CAD build for the part. Positions are in the model's coordinates, mm. Face numbers are marked on the shaded views. A direction names the side the tool comes from. Coordinates: 2 decimals unless noted, no trailing zeros. Write each loop counter-clockwise with the first axis right and the second up, starting at its lowest first coordinate (ties: lowest second). Pieces come first, ordered by that corner, then holes. Notation, with made-up numbers: (87.5, 87.25) -> (91.5, 87.25) arc R15 cw to (91.5, 113.25) -> close; hole circle Ø2 at (73, 63). An arc over 180 degrees is marked (long way). Answer as CSV lines item,"result".
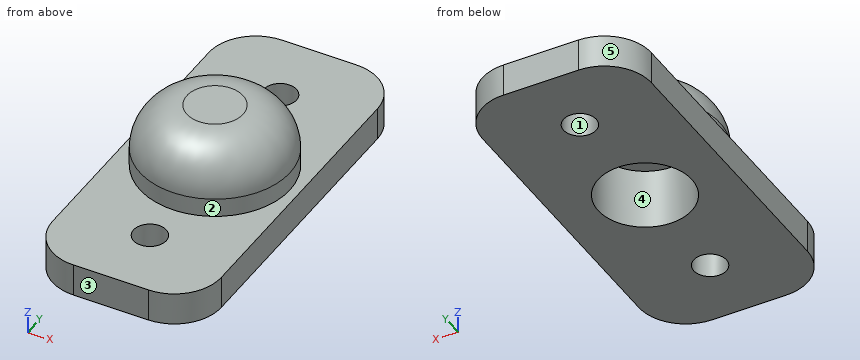
```python
from build123d import *

# Parameters (mm, degrees)
SKETCH1_W           = 18
SKETCH1_H           = 40
SKETCH1_R           = 1.75
BOSS_EXTRUDE1_DEPTH = 3.5
SKETCH2_R           = 8
BOSS_EXTRUDE2_DEPTH = 7
SKETCH3_R           = 5
CUT_EXTRUDE1_DEPTH  = 6.5
FILLET1_R           = 5


with BuildPart() as part:
    # Sketch1 → Boss-Extrude1 (new body)
    with BuildSketch(Plane.XY):
        with Locations((-6.970291657, 8.814124101)):
            Rectangle(SKETCH1_W, SKETCH1_H)
        with Locations((-6.970291657, 21.314124101)):
            Circle(SKETCH1_R, mode=Mode.SUBTRACT)
        with Locations((-6.970291657, -3.685875899)):
            Circle(SKETCH1_R, mode=Mode.SUBTRACT)
    extrude(amount=BOSS_EXTRUDE1_DEPTH)

    # Sketch2 → Boss-Extrude2 (add)
    with BuildSketch(Plane.XY.offset(3.5)):
        with Locations((-6.970291657, 8.814124101)):
            Circle(SKETCH2_R)
    extrude(amount=BOSS_EXTRUDE2_DEPTH)

    # Sketch3 → Cut-Extrude1 (cut)
    with BuildSketch(Plane(origin=(0, 0, 0), x_dir=(-1, 0, 0), z_dir=(0, 0, -1))):
        with Locations((6.970291657, 8.814124101)):
            Circle(SKETCH3_R)
    extrude(amount=-CUT_EXTRUDE1_DEPTH, mode=Mode.SUBTRACT)

    # Fillet1
    fillet1_edges = [part.edges().sort_by_distance(p)[0] for p in [
        (-14.970291657, 8.814124101, 10.5),
        (-15.970291657, 28.814124101, 1.75),
        (2.029708343, 28.814124101, 1.75),
        (2.029708343, -11.185875899, 1.75),
        (-15.970291657, -11.185875899, 1.75),
    ]]
    fillet(fillet1_edges, radius=FILLET1_R)


solid = part.part
```
Item 1: Flat gauge pins, fed straight in: pin 1 (4.5 mm diameter, centred on x = -6.97, y = -3.69, fed in from +Z); pin 2 (9 mm diameter, centred on x = -10, y = 16.5, fed in from +Z); pin 3 (1 mm diameter, centred on x = -13, z = 3.5, fed in from +Y); pin 4 (1 mm diameter, centred on y = 0.5, z = 9, fed in from -X). Where does each tip first touch, or does it go through?
Answer below:
pin 1,"stops at z = 3.5"
pin 2,"stops at z = 10.44"
pin 3,"stops at y = 28.57"
pin 4,"passes through"
Item 2: Saw through at A-A on z = 2.75. Give the cut face in (x, y), and give its area (3 significant figures).
Answer below:
outline,"(-15.97, -6.19) arc R5 ccw to (-10.97, -11.19) -> (-2.97, -11.19) arc R5 ccw to (2.03, -6.19) -> (2.03, 23.81) arc R5 ccw to (-2.97, 28.81) -> (-10.97, 28.81) arc R5 ccw to (-15.97, 23.81) -> close; hole circle Ø10 at (-6.97, 8.81); hole circle Ø3.5 at (-6.97, -3.69); hole circle Ø3.5 at (-6.97, 21.31)"
area,"601 mm2"
Item 3: Two-plate mould, pull along X, no slides. Class the marked faces 3, 4 and 5: pulls with the +X half, pulls with the -X half, needs draft (parallel to the pull), parting line crosses it, or undercut.
Answer below:
face 3,"needs draft"
face 4,"undercut"
face 5,"pulls with the -X half"
Item 4: 3-axis set-ups, long thin cutter, end or side, ignore diameter. For the marked faces 1 and 2: which of +Z, -Z, +X, -X, +Y, -Y reach the whole face in a straight line?
Answer below:
face 1,"+Z, -Z"
face 2,"+Z"
Item 5: Wall check: line 1 (Y direction, x = -6.5, z = 1.25); line 2 (Z direction, x = 0, y = 17); line 3 (Y direction, x = -8.25, z = 2). Give the ranges that are in metal, low to high. Write a range as from..to.
Answer below:
line 1,"y = -11.19..-5.37, -2..3.84, 13.79..19.63, 23..28.81"
line 2,"z = 0..3.5"
line 3,"y = -11.19..-4.88, -2.49..3.98, 13.65..20.12, 22.51..28.81"
Item 6: Saw through at B-B on x = -5.75. State how many separate pieces and enclosed holes the cut face has, and give its area (3 significant figures).
Answer below:
separate pieces,"3"
enclosed holes,"0"
area,"159 mm2"
